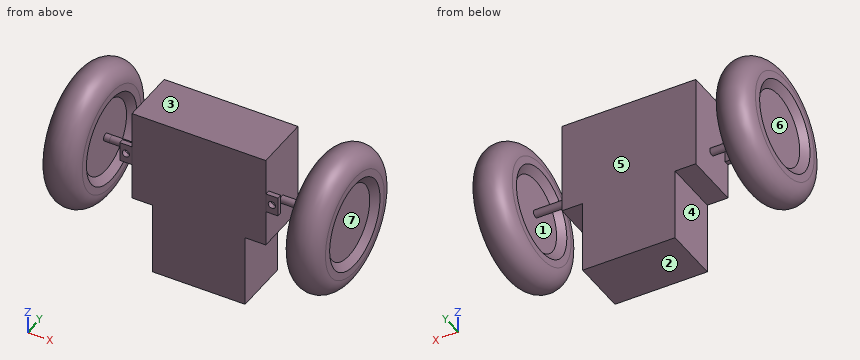
from build123d import *

# Parameters (mm, degrees)
BOSS_EXTRUDE1_DEPTH      = 11.5
BOSS_EXTRUDE1_DEPTH_BACK = 11.5
SKETCH1_W                = 55
SKETCH1_H                = 68
SKETCH2_R                = 1.5
BOSS_EXTRUDE2_DEPTH      = 15
SKETCH7_W                = 8.5
SKETCH7_H                = 30
CUT_EXTRUDE1_DEPTH       = 80.451243008
SKETCH8_W                = 5
SKETCH8_H                = 8
SKETCH8_R                = 1.5
BOSS_EXTRUDE3_DEPTH      = 2


with BuildPart() as part:
    # Sketch1 → Boss-Extrude1 (new, two sides: drawn at the far end of the back side and taken through both)
    with BuildSketch(Plane(origin=(0, 0, 0), x_dir=(1, 0, 0), z_dir=(0, 1, 0)).offset(-BOSS_EXTRUDE1_DEPTH_BACK)):
        Rectangle(SKETCH1_W, SKETCH1_H)
    extrude(amount=BOSS_EXTRUDE1_DEPTH + BOSS_EXTRUDE1_DEPTH_BACK)

    # Sketch2 → Boss-Extrude2 (add)
    with BuildSketch(Plane(origin=(27.5, 0, 0), x_dir=(0, 0, -1), z_dir=(1, 0, 0))):
        with Locations((-9, 0)):
            Circle(SKETCH2_R)
    boss_extrude2 = extrude(amount=BOSS_EXTRUDE2_DEPTH)

    # Sketch6 → Revolve1 (revolve)
    with BuildSketch(Plane(origin=(0, 0, 0), x_dir=(1, 0, 0), z_dir=(0, 1, 0)), mode=Mode.PRIVATE) as revolve1_sk:
        with BuildLine():
            Line((42.5, -7.5), (45, -7.5))
            Line((45, -7.5), (45, 6))
            Line((45, 6), (42.5, 9))
            Line((42.5, 9), (42.5, 12))
            ThreePointArc((42.5, 12), (50, 19.5), (57.5, 12))
            Line((57.5, 12), (57.5, 9))
            Line((57.5, 9), (55, 6))
            Line((55, 6), (55, -9))
            Line((55, -9), (42.5, -9))
            Line((42.5, -9), (42.5, -7.5))
        make_face()
    revolve1 = revolve(revolve1_sk.sketch.rotate(Axis((42.5, 0, 9), (1, 0, 0)), 180), axis=Axis((42.5, 0, 9), (1, 0, 0)))

    # Mirror1: Boss-Extrude2, Revolve1 across plane
    add(boss_extrude2.mirror(Plane(origin=(0, 0, 0), x_dir=(0, 0, 1), z_dir=(1, 0, 0))))
    add(revolve1.mirror(Plane(origin=(0, 0, 0), x_dir=(0, 0, 1), z_dir=(1, 0, 0))))

    # Sketch7 → Cut-Extrude1 (cut, through all)
    with BuildSketch(Plane(origin=(0, 11.5, 0), x_dir=(1, 0, 0), z_dir=(0, 1, 0))):
        with Locations((-23.25, 19)):
            Rectangle(SKETCH7_W, SKETCH7_H)
        with Locations((23.25, 19)):
            Rectangle(SKETCH7_W, SKETCH7_H)
    extrude(amount=-CUT_EXTRUDE1_DEPTH, mode=Mode.SUBTRACT)

    # Sketch8 → Boss-Extrude3 (add)
    # profile 1 of 2: a face of its own
    with BuildSketch(Plane.XZ.offset(11.5)):
        with Locations((-30, 15)):
            Rectangle(SKETCH8_W, SKETCH8_H)
        with Locations(Location((-30, 15, 0), (0, 0, 270))):
            Circle(SKETCH8_R, mode=Mode.SUBTRACT)
    # profile 2 of 2: a face of its own
    with BuildSketch(Plane.XZ.offset(11.5)):
        with Locations((30, 15)):
            Rectangle(SKETCH8_W, SKETCH8_H)
        with Locations(Location((30, 15, 0), (0, 0, 270))):
            Circle(SKETCH8_R, mode=Mode.SUBTRACT)
    extrude(amount=-BOSS_EXTRUDE3_DEPTH)


solid = part.part
Geometry: final body of the model. Coordinates: model frame, mm. Face numbers are marked on the shaded views. A direction names the side the tool comes from. Coordinates: 2 decimals unless noted, no trailing zeros. Loops run counter-clockwise (first coordinate to the right, second up) from the corner with the lowest first, then second, coordinate; pieces in that order, holes last. Notation, with made-up numbers: M 67.5,59 L 125.5,59 A19 cw 125.5,89 Z; hole C -27.75,-13.75 d1. An arc over 180 degrees is marked long. One line per item, written item: value. Start each with the question number.
1) Cut plane C-C (x = 17.5). Return loops of the section in (y, z), then the cut area to 3 significant figures.
2) Material intervals for L1, parallel to X at y = -10.5, z = 15; L2, parallel to X at y = -2, z = 22; L3, parallel to X at y = -4.5, z = 33, sorted ascending. Write a range as from..to.
3) Cut plane A-A (x = 30). Return loops of the section in (y, z).
4) Reachability of the marked faces 1, 2, 3 and 4 from +Z, -Z, +X, -X, +Y, -Y: full face, straight path, thin tool, end or side. Return the list, or none.
5) Draft query along X for the marked faces 5, 6 and 7. Return one class per face: released by +X, released by -X, zero draft, split by the parting line, or undercut.
6) Cut plane D-D (z = 20.5). Count the separate pieces of the cut face and the enclosed holes in it, then the cut area to 3 significant figures.
7) Cut plane B-B (z = -30). Return loops of the section in (x, y), then the cut area to 3 significant figures.
8) Pin query (flat end, axial travel): P1, Ø5.5, axis at x = -31, z = 14.5, coming from the +Y side; P2, Ø1.6, axis at x = -29.5, y = -10.5, coming from the -Z side; P3, Ø5, axis at x = 30, z = 15, coming from the -Y side; P4, Ø2.5, axis at x = -30, z = 15, coming from the +Y side. Return the tip coordinate at first contact, or that it passes through.
Evaluation:
1. outline: M -11.5,-34 L 11.5,-34 L 11.5,34 L -11.5,34 Z
1. area: 1,560 mm^2
2. L1: -55..-45, -32.5..-31.5, -28.5..28.5, 31.5..32.5, 45..55
2. L2: -55..-45, -27.5..27.5, 45..55
2. L3: -56.68..-43.32, -27.5..27.5, 43.32..56.68
3. outline: M -11.5,11 L -9.5,11 L -9.5,13.5 L -11.5,13.5 Z; M -11.5,16.5 L -9.5,16.5 L -9.5,19 L -11.5,19 Z; C 0,9 d3
4. face 1: none
4. face 2: -Z, +X, -X, +Y, -Y
4. face 3: +Z, +Y, -Y
4. face 4: -Z, +Y, -Y
5. face 5: undercut
5. face 6: released by -X
5. face 7: released by +X
6. separate pieces: 3
6. enclosed holes: 0
6. area: 2,490 mm^2
7. outline: M -19,-11.5 L 19,-11.5 L 19,11.5 L -19,11.5 Z
7. area: 874 mm^2
8. P1: y = -9.5
8. P2: z = 11
8. P3: y = -11.5
8. P4: through
